from build123d import *

# Parameters (mm, degrees)
EXTRUDE_1_DEPTH      = 10
EXTRUDE_1_DEPTH_BACK = 20
EXTRUDE_1_2_DEPTH    = 30


with BuildPart() as part:
    # 草图1 → Extrude 1 (new, two sides: drawn at the far end of the back side and taken through both)
    with BuildSketch(Plane.XY.offset(-EXTRUDE_1_DEPTH_BACK)):
        with BuildLine():
            Line((0, 13.930688276), (50.29066082, 13.930688276))
            ThreePointArc((50.29066082, 13.930688276), (64.221349097, 0), (50.29066082, -13.930688276))
            Line((50.29066082, -13.930688276), (0, -13.930688276))
            ThreePointArc((0, -13.930688276), (-13.930688276, 0), (0, 13.930688276))
        make_face()
    extrude(amount=EXTRUDE_1_DEPTH + EXTRUDE_1_DEPTH_BACK)

    # 草图7 → Extrude 1 2 (add)
    with BuildSketch(Plane.XY.offset(10)):
        with BuildLine():
            Line((50.29066082, 13.930688276), (0, 13.930688276))
            ThreePointArc((0, 13.930688276), (-13.930688276, 0), (0, -13.930688276))
            Line((0, -13.930688276), (50.29066082, -13.930688276))
            ThreePointArc((50.29066082, -13.930688276), (64.221349097, 0), (50.29066082, 13.930688276))
        make_face()
        with BuildLine():
            Line((50.29066082, 8.930688276), (0, 8.930688276))
            ThreePointArc((0, 8.930688276), (-8.930688276, 0), (0, -8.930688276))
            Line((0, -8.930688276), (50.29066082, -8.930688276))
            ThreePointArc((50.29066082, -8.930688276), (59.221349097, 0), (50.29066082, 8.930688276))
        make_face(mode=Mode.SUBTRACT)
    extrude(amount=EXTRUDE_1_2_DEPTH)


solid = part.part
Source: CAD feature listing. Evaluate the final solid. Frame: model axes, mm. A direction names the side the tool comes from. Round coordinates to 2 decimals unless told otherwise and drop trailing zeros. Write each loop counter-clockwise with the first axis right and the second up, starting at its lowest first coordinate (ties: lowest second). Pieces come first, ordered by that corner, then holes. Notation, with made-up numbers: M -32.5,49 L -22.5,49 A25 cw -22.5,74 Z; hole C 29,-35.75 d2. An arc over 180 degrees is marked long. One line per item, written item: value. Start each with the question number.
Item 1: Pin query (flat end, axial travel): pin 1 (9 mm diameter, centred on x = 30, y = 0, fed in from +Z); pin 2 (2 mm diameter, centred on y = 8.5, z = 6, fed in from -X); pin 3 (10 mm diameter, centred on y = -4.5, z = 33.5, fed in from +X); pin 4 (3 mm diameter, centred on y = 7.5, z = 3.5, fed in from +X). Return the tip coordinate at first contact, or that it passes through.
Item 2: Section query B-B (x = 19). Return the cut outline in (y, z).
Item 3: Set-up query: faces 4 (the flat face through (25, 8.931, 25)), 5 (the flat face through (26, 0, -20)). Return all of +Z, -Z, +X, -X, +Y, -Y with unobstructed straight access to the full face (end or side cutting, diameter ignored); none if empty.
Item 4: Section query A-A (z = 18.5). Return the cut outline in (x, y), plus the area to 3 significant figures.
Item 5: Section query D-D (z = 7.5). Return the cut outline in (x, y), plus the area to 3 significant figures.
Item 6: Ray query, L1, parallel to Y at x = 47.5, z = 25.5; L2, parallel to Z at x = 43, y = -6.25; L3, parallel to X at y = -0.25, z = 5. Return the intervals inside material, ascending. Write a range as from..to.
Item 7: Mould query, pull axis X, two halves, no side actions, for faces 1 (the flat face through (26, 0, 10)), 2 (the cylindrical face through (64.218, -0.306, 9.58)), 3 (the cylindrical face through (-13.927, 0.306, 9.58)). Classes: pulls with the +X half, pulls with the -X half, needs draft (parallel to the pull), parting line crosses it, or undercut.
Item 8: Section query C-C (y = 0). Return the cut outline in (x, z), plus the area to 3 significant figures.
Result set:
1. pin 1: stops at z = 10
1. pin 2: stops at x = -11.74
1. pin 3: stops at x = 64.22
1. pin 4: stops at x = 62.86
2. outline: M -13.93,-20 L 13.93,-20 L 13.93,40 L 8.93,40 L 8.93,10 L -8.93,10 L -8.93,40 L -13.93,40 Z
3. face 4: +Z
3. face 5: -Z, +X, -X, +Y, -Y
4. outline: M 0,-13.93 L 50.29,-13.93 A13.93 ccw 50.29,13.93 L 0,13.93 A13.93 ccw Z; hole M 0,-8.93 L 50.29,-8.93 A8.93 ccw 50.29,8.93 L 0,8.93 A8.93 ccw Z
4. area: 862 mm²
5. outline: M 0,-13.93 L 50.29,-13.93 A13.93 ccw 50.29,13.93 L 0,13.93 A13.93 ccw Z
5. area: 2,010 mm²
6. L1: y = -13.93..-8.93, 8.93..13.93
6. L2: z = -20..10
6. L3: x = -13.93..64.22
7. face 1: undercut
7. face 2: pulls with the +X half
7. face 3: pulls with the -X half
8. outline: M -13.93,-20 L 64.22,-20 L 64.22,40 L 59.22,40 L 59.22,10 L -8.93,10 L -8.93,40 L -13.93,40 Z
8. area: 2,640 mm²
